Work out the finished part from the listing and answer in its coordinate system (mm). A direction names the side the tool comes from. Give positions to 0.01 mm unless a question says otherwise; leave off trailing zeros. Loops run counter-clockwise (first coordinate to the right, second up) from the corner with the lowest first, then second, coordinate; pieces in that order, holes last. Notation, with made-up numbers: M -3.75,83.25 L 40.25,83.25 A27 cw 40.25,102.25 Z; hole C 4.5,52 d6. An arc over 180 degrees is marked long. Answer as a JSON object with one key per item and string values. Group by question number.
```python
from build123d import *

# Parameters (mm, degrees)
SKETCH1_W                                     = 60.325
SKETCH1_H                                     = 25.4
BOSS_EXTRUDE1_DEPTH                           = 18.415
SKETCH2_W                                     = 41.275
SKETCH2_H                                     = 24.13
CUT_EXTRUDE1_DEPTH                            = 44.520669012
SKETCH3_W                                     = 12.7
SKETCH3_H                                     = 36.83
CUT_EXTRUDE2_DEPTH                            = 9.525
SKETCH4_W                                     = 6.35
SKETCH4_H                                     = 6.35
CUT_EXTRUDE3_DEPTH                            = 3.175
SKETCH5_R                                     = 1.5875
CUT_EXTRUDE4_DEPTH                            = 3.175
F_8_32_TAPPED_HOLE1_D                         = 3.4544
F_8_32_TAPPED_HOLE2_D                         = 3.4544
CBORE_START                                   = -18.415
CBORE_SLOT_FOR_8_SOCKET_HEAD_CAP_SCREW1_DEPTH = 12.7
CBORE_SLOT_FOR_8_SOCKET_HEAD_CAP_SC_3_DEPTH   = 4.1656


# Read off the part's stored shape, not the designer's step: CBORE SLOT for #8 Socket Head Cap Screw1
with BuildPart() as part:
    # Sketch1 → Boss-Extrude1 (new, symmetric)
    with BuildSketch(Plane(origin=(0, 0, 0), x_dir=(1, 0, 0), z_dir=(0, 1, 0))):
        Rectangle(SKETCH1_W, SKETCH1_H)
    extrude(amount=BOSS_EXTRUDE1_DEPTH, both=True)

    # Sketch2 → Cut-Extrude1 (cut, through all)
    with BuildSketch(Plane.XY.offset(12.7)):
        with Locations((0, 6.35)):
            Rectangle(SKETCH2_W, SKETCH2_H)
    extrude(amount=-CUT_EXTRUDE1_DEPTH, mode=Mode.SUBTRACT)

    # Sketch3 → Cut-Extrude2 (cut)
    with BuildSketch(Plane(origin=(30.1625, 0, 0), x_dir=(0, 0, -1), z_dir=(1, 0, 0))):
        with Locations((-6.35, 0)):
            Rectangle(SKETCH3_W, SKETCH3_H)
    cut_extrude2 = extrude(amount=-CUT_EXTRUDE2_DEPTH, mode=Mode.SUBTRACT)

    # Sketch4 → Cut-Extrude3 (cut)
    with BuildSketch(Plane.XY):
        with Locations((26.9875, 15.24)):
            Rectangle(SKETCH4_W, SKETCH4_H)
    cut_extrude3 = extrude(amount=-CUT_EXTRUDE3_DEPTH, mode=Mode.SUBTRACT)

    # Sketch5 → Cut-Extrude4 (cut)
    with BuildSketch(Plane.XY):
        with Locations((23.8125, 12.065)):
            Circle(SKETCH5_R)
    cut_extrude4 = extrude(amount=-CUT_EXTRUDE4_DEPTH, mode=Mode.SUBTRACT)

    # #8-32 Tapped Hole1 (through all)
    with Locations(Plane.XY):
        with Locations((26.9875, 6.985)):
            f_8_32_tapped_hole1 = Hole(F_8_32_TAPPED_HOLE1_D / 2)

    # Mirror1: Cut-Extrude2, Cut-Extrude3, Cut-Extrude4, #8-32 Tapped Hole1 across plane
    add(cut_extrude2.mirror(Plane(origin=(0, 0, 0), x_dir=(0, 0, 1), z_dir=(1, 0, 0))), mode=Mode.SUBTRACT)
    add(cut_extrude3.mirror(Plane(origin=(0, 0, 0), x_dir=(0, 0, 1), z_dir=(1, 0, 0))), mode=Mode.SUBTRACT)
    add(cut_extrude4.mirror(Plane(origin=(0, 0, 0), x_dir=(0, 0, 1), z_dir=(1, 0, 0))), mode=Mode.SUBTRACT)
    add(f_8_32_tapped_hole1.mirror(Plane(origin=(0, 0, 0), x_dir=(0, 0, 1), z_dir=(1, 0, 0))), mode=Mode.SUBTRACT)

    # #8-32 Tapped Hole2 (through all)
    with Locations(Plane(origin=(0, -18.415, 0), x_dir=(-1, 0, 0), z_dir=(0, -1, 0))):
        with Locations((16.51, 0)):
            f_8_32_tapped_hole2 = Hole(F_8_32_TAPPED_HOLE2_D / 2)

    # CBORE SLOT for _8 Socket Head Cap Sc 2 → CBORE SLOT for #8 Socket Head Cap Screw1 (cut)
    with BuildSketch(Plane(origin=(0, 0, 0), x_dir=(1, 0, 0), z_dir=(0, 1, 0)).offset(CBORE_START)):
        with BuildLine():
            ThreePointArc((-9.652, 4.7371), (-7.4041, 6.985), (-9.652, 9.2329))
            Line((-9.652, 9.2329), (-10.668, 9.2329))
            ThreePointArc((-10.668, 9.2329), (-12.9159, 6.985), (-10.668, 4.7371))
            Line((-10.668, 4.7371), (-9.652, 4.7371))
        make_face()
        with BuildLine():
            ThreePointArc((9.652, 9.2329), (7.4041, 6.985), (9.652, 4.7371))
            Line((9.652, 4.7371), (10.668, 4.7371))
            ThreePointArc((10.668, 4.7371), (12.9159, 6.985), (10.668, 9.2329))
            Line((10.668, 9.2329), (9.652, 9.2329))
        make_face()
        with BuildLine():
            ThreePointArc((6.858, -9.2329), (9.1059, -6.985), (6.858, -4.7371))
            Line((6.858, -4.7371), (5.842, -4.7371))
            ThreePointArc((5.842, -4.7371), (3.5941, -6.985), (5.842, -9.2329))
            Line((5.842, -9.2329), (6.858, -9.2329))
        make_face()
        with BuildLine():
            ThreePointArc((-6.858, -4.7371), (-9.1059, -6.985), (-6.858, -9.2329))
            Line((-6.858, -9.2329), (-5.842, -9.2329))
            ThreePointArc((-5.842, -9.2329), (-3.5941, -6.985), (-5.842, -4.7371))
            Line((-5.842, -4.7371), (-6.858, -4.7371))
        make_face()
    extrude(amount=CBORE_SLOT_FOR_8_SOCKET_HEAD_CAP_SCREW1_DEPTH, mode=Mode.SUBTRACT)

    # CBORE SLOT for _8 Socket Head Cap Sc 3 o → CBORE SLOT for _8 Socket Head Cap Sc 3 (cut)
    # profile 1 of 4: a face of its own
    with BuildSketch(Plane(origin=(0, 0, 0), x_dir=(1, 0, 0), z_dir=(0, 1, 0)).offset(CBORE_START)):
        with BuildLine():
            ThreePointArc((-9.652, 3.01625), (-5.68325, 6.985), (-9.652, 10.95375))
            Line((-9.652, 10.95375), (-10.668, 10.95375))
            ThreePointArc((-10.668, 10.95375), (-14.63675, 6.985), (-10.668, 3.01625))
            Line((-10.668, 3.01625), (-9.652, 3.01625))
        make_face()
        with BuildLine():
            Line((-10.668, 9.2329), (-9.652, 9.2329))
            ThreePointArc((-9.652, 9.2329), (-7.4041, 6.985), (-9.652, 4.7371))
            Line((-9.652, 4.7371), (-10.668, 4.7371))
            ThreePointArc((-10.668, 4.7371), (-12.9159, 6.985), (-10.668, 9.2329))
        make_face(mode=Mode.SUBTRACT)
    # profile 2 of 4: a face of its own
    with BuildSketch(Plane(origin=(0, 0, 0), x_dir=(1, 0, 0), z_dir=(0, 1, 0)).offset(CBORE_START)):
        with BuildLine():
            ThreePointArc((9.652, 10.95375), (5.68325, 6.985), (9.652, 3.01625))
            Line((9.652, 3.01625), (10.668, 3.01625))
            ThreePointArc((10.668, 3.01625), (14.63675, 6.985), (10.668, 10.95375))
            Line((10.668, 10.95375), (9.652, 10.95375))
        make_face()
        with BuildLine():
            Line((10.668, 4.7371), (9.652, 4.7371))
            ThreePointArc((9.652, 4.7371), (7.4041, 6.985), (9.652, 9.2329))
            Line((9.652, 9.2329), (10.668, 9.2329))
            ThreePointArc((10.668, 9.2329), (12.9159, 6.985), (10.668, 4.7371))
        make_face(mode=Mode.SUBTRACT)
    # profile 3 of 4: a face of its own
    with BuildSketch(Plane(origin=(0, 0, 0), x_dir=(1, 0, 0), z_dir=(0, 1, 0)).offset(CBORE_START)):
        with BuildLine():
            ThreePointArc((6.858, -10.95375), (10.82675, -6.985), (6.858, -3.01625))
            Line((6.858, -3.01625), (5.842, -3.01625))
            ThreePointArc((5.842, -3.01625), (1.87325, -6.985), (5.842, -10.95375))
            Line((5.842, -10.95375), (6.858, -10.95375))
        make_face()
        with BuildLine():
            Line((5.842, -4.7371), (6.858, -4.7371))
            ThreePointArc((6.858, -4.7371), (9.1059, -6.985), (6.858, -9.2329))
            Line((6.858, -9.2329), (5.842, -9.2329))
            ThreePointArc((5.842, -9.2329), (3.5941, -6.985), (5.842, -4.7371))
        make_face(mode=Mode.SUBTRACT)
    # profile 4 of 4: a face of its own
    with BuildSketch(Plane(origin=(0, 0, 0), x_dir=(1, 0, 0), z_dir=(0, 1, 0)).offset(CBORE_START)):
        with BuildLine():
            ThreePointArc((-6.858, -3.01625), (-10.82675, -6.985), (-6.858, -10.95375))
            Line((-6.858, -10.95375), (-5.842, -10.95375))
            ThreePointArc((-5.842, -10.95375), (-1.87325, -6.985), (-5.842, -3.01625))
            Line((-5.842, -3.01625), (-6.858, -3.01625))
        make_face()
        with BuildLine():
            Line((-5.842, -9.2329), (-6.858, -9.2329))
            ThreePointArc((-6.858, -9.2329), (-9.1059, -6.985), (-6.858, -4.7371))
            Line((-6.858, -4.7371), (-5.842, -4.7371))
            ThreePointArc((-5.842, -4.7371), (-3.5941, -6.985), (-5.842, -9.2329))
        make_face(mode=Mode.SUBTRACT)
    extrude(amount=CBORE_SLOT_FOR_8_SOCKET_HEAD_CAP_SC_3_DEPTH, mode=Mode.SUBTRACT)

    # Mirror2: #8-32 Tapped Hole2 across plane
    add(f_8_32_tapped_hole2.mirror(Plane(origin=(0, 0, 0), x_dir=(0, 0, 1), z_dir=(1, 0, 0))), mode=Mode.SUBTRACT)


solid = part.part
```
Item 1: For a pull along X with two mould halves and no side action, classify faces 5 (the cylindrical face through (14.636, -16.361, -6.898)), 6 (the flat face through (-25, 18.415, -8)), 7 (the flat face through (30.162, 0, -6)), 8 (the flat face through (-30.162, 0, -6)) as pulls with the +X half, pulls with the -X half, needs draft (parallel to the pull), parting line crosses it, or undercut.
Item 2: A tool of negligible diameter and unlimited length cuts with its end or side. For faces 1 (the cylindrical face through (22.654, 10.98, -1.565)), 2 (the flat face through (25, -4, 0)), 3 (the flat face through (-20.638, 6, -6)), 4 (the cylindrical face through (1.874, -16.361, 6.898)), from which of +Z, -Z, +X, -X, +Y, -Y can it reach the whole face along a straight path? Write none if from no direction.
Item 3: A cutting plane is placed at D-D (y = -11.5). Determine the outline of the cut face in (x, z) (1 decimal).
Item 4: A cutting plane is placed at A-A (x = 16.51). Determine the outline of the cut face in (y, z) (3 decimals), and give its area (3 significant figures).
Item 5: A cutting plane is placed at B-B (y = -1). Determine the outline of the cut face in (x, z).
Item 6: Find the intervals of material crossed by probe 1 along X at (y, z) = (-11, -6.75); probe 2 along X at (y, z) = (-10, -0.75); probe 3 along X at (y, z) = (-3, -9), in increasing order. Write a range as [from, to].
Item 7: A cutting plane is placed at C-C (z = 5.5). Determine the outline of the cut face in (x, y) (1 decimal).
Item 8: Given pin 1 Ø7.5 at (x, y) = (23, -2.5) entering from +Z; pin 2 Ø1 at (y, z) = (16, -1.5) entering from -X; pin 3 Ø2.5 at (x, y) = (-23.81, 12.06) entering from +Z (3 decimals), each flat-ended and moving along its own axis, determine where each tip first touches the part or whether it passes through.
The answers:
{
 "1": {"face 5": "undercut", "face 6": "needs draft", "face 7": "pulls with the +X half", "face 8": "pulls with the -X half"},
 "2": {"face 1": "+Z", "face 2": "+Z, +X, +Y, -Y", "face 3": "+Z, -Z, +Y", "face 4": "-Y"},
 "3": {"outline": "M -30.2,-12.7 L 30.2,-12.7 L 30.2,0 L 20.6,0 L 20.6,12.7 L -20.6,12.7 L -20.6,0 L -30.2,0 Z; hole C -16.5,0 d3.5; hole M -10.7,-9.2 L -9.7,-9.2 A2.2 ccw -9.7,-4.7 L -10.7,-4.7 A2.2 ccw Z; hole M -6.9,4.7 L -5.8,4.7 A2.2 ccw -5.8,9.2 L -6.9,9.2 A2.2 ccw Z; hole M 5.8,4.7 L 6.9,4.7 A2.2 ccw 6.9,9.2 L 5.8,9.2 A2.2 ccw Z; hole M 9.7,-9.2 L 10.7,-9.2 A2.2 ccw 10.7,-4.7 L 9.7,-4.7 A2.2 ccw Z; hole C 16.5,0 d3.5"},
 "4": {"outline": "M -18.415,-12.7 L -5.715,-12.7 L -5.715,-1.727 L -18.415,-1.727 Z; M -18.415,1.727 L -5.715,1.727 L -5.715,12.7 L -18.415,12.7 Z", "area": "279 mm^2"},
 "5": {"outline": "M -30.16,-12.7 L -20.64,-12.7 L -20.64,0 L -30.16,0 Z; M 20.64,-12.7 L 30.16,-12.7 L 30.16,0 L 20.64,0 Z"},
 "6": {"probe 1": "x = [-30.16, -12.9], [-7.42, 7.42], [12.9, 30.16]", "probe 2": "x = [-30.16, -18.07], [-14.95, 14.95], [18.07, 30.16]", "probe 3": "x = [-30.16, -20.64], [20.64, 30.16]"},
 "7": {"outline": "M -20.6,-18.4 L -10.5,-18.4 L -10.5,-14.2 L -8.5,-14.2 L -8.5,-5.7 L -20.6,-5.7 Z; M -4.2,-14.2 L -2.2,-14.2 L -2.2,-18.4 L 2.2,-18.4 L 2.2,-14.2 L 4.2,-14.2 L 4.2,-5.7 L -4.2,-5.7 Z; M 8.5,-14.2 L 10.5,-14.2 L 10.5,-18.4 L 20.6,-18.4 L 20.6,-5.7 L 8.5,-5.7 Z"},
 "8": {"pin 1": "stops at z = 0", "pin 2": "stops at x = -23.81", "pin 3": "stops at z = -3.175"}
}
